Input: part model. Units: mm. Frame: model coordinates. A direction names the side the tool comes from. Coordinates: 2 decimals unless noted, no trailing zeros. Write each loop counter-clockwise with the first axis right and the second up, starting at its lowest first coordinate (ties: lowest second). Pieces come first, ordered by that corner, then holes.
Autodesk Inventor part; units mm, degrees
ref_plane "YZ Plane" through (0, 0, 0) normal (1, 0, 0) x (0, 1, 0)
ref_plane "XZ Plane" through (0, 0, 0) normal (0, 1, 0) x (-1, 0, 0)
ref_plane "XY Plane" through (0, 0, 0) normal (0, 0, 1) x (1, 0, 0)
sketch "草圖1" plane through (0, 0, 0) normal (0, 0, 1) x (1, 0, 0)
  line L0 (0, 0) -> (12, 0)
  line L1 (12, 0) -> (16, -4.5023)
  line L2 (16, -4.5023) -> (0, -4.5023)
  line L3 (0, 0) -> (0, -4.5023)
  dimension "d0" = 12
  dimension "d1" = 16
revolve "迴轉1" add sketch "草圖1" angle 360 about axis through (0, 0, 0) along (0, -1, 0)
sketch "草圖2" plane through (0, -4.5023, 0) normal (0, -1, 0) x (1, 0, 0)
  circle A0 centre (0, 0) radius 17
  dimension "d3" = 34
extrude "擠出1" add sketch "草圖2" along normal blind 6
sketch "草圖3" plane through (0, -10.5023, 0) normal (0, -1, 0) x (1, 0, 0)
  circle A0 centre (0, 0) radius 16
  circle A1 centre (0, 0) radius 16
  line L0 (0, 16) -> (0, -16)
  dimension "d6" = 32
revolve "迴轉2" add sketch "草圖3" angle 180 about axis through (0, -10.5023, 16) along (0, 0, -1) picked at (2.314, 4.8052) contours A0 L0
sketch "草圖4" plane through (0, 0, 0) normal (0, 0, 1) x (1, 0, 0)
  arc A0 (-16, -10.5023) -> (16, -10.5023) centre (0, -10.5023) ccw
  arc A1 (-16, -10.5023) -> (16, -10.5023) centre (0, -10.5023) ccw
  line L0 (-17, -10.5023) -> (17, -10.5023)
  arc A2 (-15, -10.5023) -> (15, -10.5023) centre (0, -10.5023) ccw
  line L1 (-16, -10.5023) -> (-15, -10.5023)
  line L2 (15, -10.5023) -> (16, -10.5023)
  point P0 (0, 0)
  dimension "d8" = 1
extrude "擠出2" cut sketch "草圖4" along normal mid plane 1 contours L0 A2 A0
sketch "草圖5" plane through (0, 0, 0) normal (1, 0, 0) x (0, 1, 0)
  arc A0 (-10.5023, 16) -> (-26.4945, 0.5) centre (-10.5023, 0) ccw
  arc A1 (-26.4945, -0.5) -> (-10.5023, -16) centre (-10.5023, 0) ccw
  arc A2 (-10.5023, 16) -> (-10.5023, -16) centre (-10.5023, 0) ccw
  line L0 (-10.5023, -16) -> (-10.5023, -0.5)
  arc A3 (-10.5023, 15) -> (-10.5023, -15) centre (-10.5023, 0) ccw
  line L1 (-10.5023, -16) -> (-10.5023, -15)
  line L2 (-10.5023, 16) -> (-10.5023, 15)
  line L3 (-10.5023, 17) -> (-10.5023, -17)
  point P0 (0, 0)
  point P1 (-26.4945, 0.5)
  point P2 (-26.4945, -0.5)
  dimension "d11" = 1
extrude "擠出3" cut sketch "草圖5" along normal mid plane 1 contours L2 A3 L0 A1 A2 A0
sketch "草圖6" plane through (0, 0, 0) normal (0, 1, 0) x (1, 0, 0)
  line L0 (0.5, -0.5) -> (0, 0)
  circle A0 centre (0, 0) radius 4
  dimension "d14" = 8
extrude "擠出4" add sketch "草圖6" against normal blind 30
properties part number "屋1 物1 base"
Item 1: Section query D-D, the plane y = -16. Return loops of the section in (x, z).
Item 2: Access query for faces 1 (the face through (0, 0, 0)), 2 (the face through (-11.84, -19.71, -0.01)), 3 (the face through (12, -20, -0.5)), 4 (the face through (9.139, -7.46, -14.334)), 5 (the face through (13, -4.502, -10)). Directions: +Z, -Z, +X, -X, +Y, -Y. A direction counts if a zero-diameter tool reaches every point of the face in a straight line with its end or side. Return the directions, or none.
Item 3: Section query A-A, the plane z = 0. Return loops of the section in (x, y).
Item 4: Pull-direction query (Z, two-part tool) for faces 6 (the face through (-0.01, -19.71, 11.84)), 7 (the face through (0, -19.5, -12)), 8 (the face through (-12, -20, 0.5)); classes: released by +Z, released by -Z, zero draft, split by the parting line, or undercut.
Item 5: Pin query (flat end, axial travel): pin 1 Ø1 at (y, z) = (-16.5, -11) entering from +X; pin 2 Ø13 at (x, y) = (11.5, -18) entering from +Z; pin 3 Ø9.5 at (x, y) = (-8, -15.5) entering from -Z. Return the tip coordinate at first contact, or that it passes through.
Item 6: Section query C-C, the plane y = -27. Return loops of the section in (x, z).
Item 7: Material intervals for line 1 (Y direction, x = -7, z = 15); line 2 (X direction, y = -17, z = 11); line 3 (Z direction, x = 7.5, y = -17.5), sorted ascending.
Item 8: Section query B-B, the plane y = -11.5. Return loops of the section in (x, z), then the cut area to 3 significant figures.
The answers:
1. outline: (-15.02, -0.5) arc R15.03 ccw to (-0.5, -15.02) - (-0.5, -13.96) - (0.5, -13.96) - (0.5, -15.02) arc R15.03 ccw to (15.02, -0.5) - (13.96, -0.5) - (13.96, 0.5) - (15.02, 0.5) arc R15.03 ccw to (0.5, 15.02) - (0.5, 13.96) - (-0.5, 13.96) - (-0.5, 15.02) arc R15.03 ccw to (-15.02, 0.5) - (-13.96, 0.5) - (-13.96, -0.5) - close
2. face 1: +Z, -Z, +X, -X, +Y
2. face 2: -X, -Y
2. face 3: +X, -Y
2. face 4: +Y, -Y
2. face 5: +Y
3. outline: (-17, -10.5) - (-15, -10.5) arc R15 ccw to (-4, -24.96) - (-4, -30) - (4, -30) - (4, -24.96) arc R15 ccw to (15, -10.5) - (17, -10.5) - (17, -4.5) - (16, -4.5) - (12, 0) - (-12, 0) - (-16, -4.5) - (-17, -4.5) - close
4. face 6: released by +Z
4. face 7: released by -Z
4. face 8: undercut
5. pin 1: stops at x = 10.55
5. pin 2: stops at z = 14.27
5. pin 3: stops at z = -15.3
6. outline: circle Ø8 at (0, 0)
7. line 1: y = -10.5 to -4.5
7. line 2: x = -9.63 to 9.63
7. line 3: z = -12.28 to 12.28
8. outline: (-15.96, -0.5) arc R15.97 ccw to (-0.5, -15.96) - (-0.5, -14.97) - (0.5, -14.97) - (0.5, -15.96) arc R15.97 ccw to (15.96, -0.5) - (14.97, -0.5) - (14.97, 0.5) - (15.96, 0.5) arc R15.97 ccw to (0.5, 15.96) - (0.5, 14.97) - (-0.5, 14.97) - (-0.5, 15.96) arc R15.97 ccw to (-15.96, 0.5) - (-14.97, 0.5) - (-14.97, -0.5) - close
8. area: 797 mm2
